Source: CAD feature listing. Evaluate the final solid. Frame: model axes, mm. Face numbers are marked on the shaded views. A direction names the side the tool comes from. Give positions to 0.01 mm unless a question says otherwise; leave off trailing zeros. Write each loop counter-clockwise with the first axis right and the second up, starting at its lowest first coordinate (ties: lowest second). Pieces come first, ordered by that corner, then holes. Notation, with made-up numbers: (-9, -34) - (11, -34) arc R35 cw to (11, 5) - close; hole circle Ø9 at (32, 43.25). An arc over 180 degrees is marked (long way). One line per question, with ' | ' between items. Start each with the question number.
(1) Access query for the marked faces 1 and 2. Directions: +Z, -Z, +X, -X, +Y, -Y. A direction counts if a zero-diameter tool reaches every point of the face in a straight line with its end or side. Return the directions, or none.
(2) Pin query (flat end, axial travel): pin 1 (1.5 mm diameter, centred on x = 10, z = -1, fed in from -Y). Return the tip coordinate at first contact, or that it passes through.
(3) Section A-A, the plane x = 10.75. Return loops of the section in (y, z), plus the area to 3 significant figures.
(4) Ray query, line 1 (Y direction, x = 12, z = -0.1); line 2 (X direction, y = 1, z = 1.75); line 3 (Z direction, x = 4, y = -1). Return the intervals inside material, ascending. Write a range as [from, to].
Solid Edge part; units mm, degrees
sketch "Sketch1" plane through (0, 0, 0) normal (0, 0, 1) x (1, 0, 0)
  line L0 (0, 0) -> (0, 2.15)
  line L1 (0, 2.15) -> (0.25, 2.15)
  line L2 (0.25, 2.15) -> (1.0657, 1.3343)
  arc A0 (1.0657, 1.3343) -> (1.6314, 1.1) centre (1.6314, 1.9) ccw
  line L3 (1.6314, 1.1) -> (17.5, 1.1)
  line L4 (17.5, 1.1) -> (19, 0)
  line L5 (19, 0) -> (0, 0)
revolve "RevolvedProtrusion1" add sketch "Sketch1" angle 360 about axis through (23.3, 0, 0) along (-1, 0, 0)
cosmetic_thread "Thread_1" thread depth 15.4
sketch "Sketch2" plane through (0, 0, 0) normal (1, 0, 0) x (0, 1, 0)
  line L0 (0.2375, 0.95) -> (-0.2375, 0.95)
  line L1 (-0.2375, 0.95) -> (-0.1876, 0.38)
  line L2 (-0.1876, 0.38) -> (-0.2375, 0.2375)
  line L3 (-0.2375, 0.2375) -> (-0.38, 0.1876)
  line L4 (-0.38, 0.1876) -> (-0.95, 0.2375)
  line L5 (-0.95, 0.2375) -> (-0.95, -0.2375)
  line L6 (-0.95, -0.2375) -> (-0.38, -0.1876)
  line L7 (-0.38, -0.1876) -> (-0.2375, -0.2375)
  line L8 (-0.2375, -0.2375) -> (-0.1876, -0.38)
  line L9 (-0.1876, -0.38) -> (-0.2375, -0.95)
  line L10 (-0.2375, -0.95) -> (0.2375, -0.95)
  line L11 (0.2375, -0.95) -> (0.1876, -0.38)
  line L12 (0.1876, -0.38) -> (0.2375, -0.2375)
  line L13 (0.2375, -0.2375) -> (0.38, -0.1876)
  line L14 (0.38, -0.1876) -> (0.95, -0.2375)
  line L15 (0.95, -0.2375) -> (0.95, 0.2375)
  line L16 (0.95, 0.2375) -> (0.38, 0.1876)
  line L17 (0.38, 0.1876) -> (0.2375, 0.2375)
  line L18 (0.2375, 0.2375) -> (0.1876, 0.38)
  line L19 (0.1876, 0.38) -> (0.2375, 0.95)
extrude "ExtrudedCutout_1" cut sketch "Sketch2" along normal blind 0.7273
properties part number "bene_inox_212409-2,2X19"
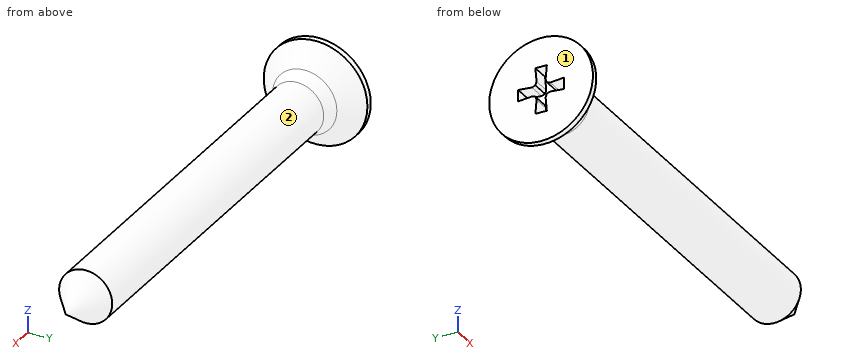
Check sheet entries:
1) face 1: +Z, -Z, -X, +Y, -Y | face 2: +X
2) pin 1: y = -1.07
3) outline: circle Ø2.2 at (0, 0) | area: 3.80 mm²
4) line 1: [-1.1, 1.1] | line 2: [0, 0.38] | line 3: [-0.46, 0.46]
